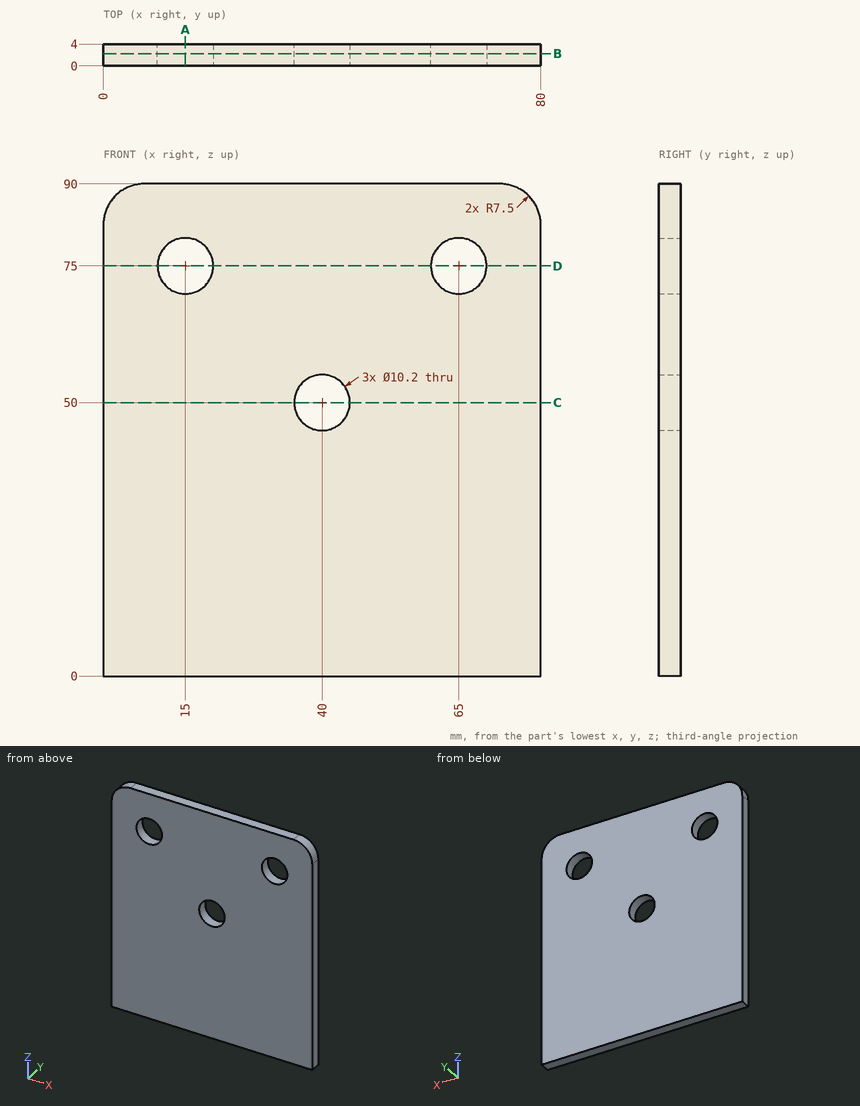
Job drawing, mm, ordinate dimensions from the low corner. One solid piece. Give positions to 0.01 mm unless a question says otherwise; leave off trailing zeros. Order: outer loops, then holes, each group sorted by start corner. A loop starts at its lowest first (then second) coordinate and runs counter-clockwise, first axis right, second up. Notation, with made-up numbers: (80, 69) - (135, 69) arc R23 cw to (135, 85) - close; hole circle Ø5 at (57, 34). An arc over 180 degrees is marked (long way). Return JSON: item names as keys, results as strings.
1) Probe line 1 (Z direction, x = 40, y = 2.1); line 2 (Z direction, x = 65, y = 0.95); line 3 (Z direction, x = 73, y = 0.75). List the from-to ranges inside material, lowest first. Write a range as from..to.
Geometry says:
{"line 1": "0..44.9, 55.1..90", "line 2": "0..69.9, 80.1..90", "line 3": "0..89.98"}
2) Cut at C-C, the plane z = 50. Give the cut face in (x, y).
Geometry says:
{"outline": "(0, 0) - (34.9, 0) - (34.9, 4) - (0, 4) - close; (45.1, 0) - (80, 0) - (80, 4) - (45.1, 4) - close"}
3) Cut at A-A, the plane x = 15. Give the cut face in (y, z), plus the area to 3 significant figures.
Geometry says:
{"outline": "(0, 0) - (4, 0) - (4, 69.9) - (0, 69.9) - close; (0, 80.1) - (4, 80.1) - (4, 90) - (0, 90) - close", "area": "319 mm²"}
4) Flat gauge pin, fed straight in: P1, Ø9, axis at x = 65, z = 75, coming from the -Y side. Where does the tip first touch, or does it go through?
Geometry says:
{"P1": "through"}
5) Cut at D-D, the plane z = 75. Give the cut face in (x, y), plus the area to 3 significant figures.
Geometry says:
{"outline": "(0, 0) - (9.9, 0) - (9.9, 4) - (0, 4) - close; (20.1, 0) - (59.9, 0) - (59.9, 4) - (20.1, 4) - close; (70.1, 0) - (80, 0) - (80, 4) - (70.1, 4) - close", "area": "238 mm²"}
6) Cut at B-B, the plane y = 2.25. Give the cut face in (x, z), plus the area to 3 significant figures.
Geometry says:
{"outline": "(0, 0) - (80, 0) - (80, 82.5) arc R7.5 ccw to (72.5, 90) - (7.5, 90) arc R7.5 ccw to (0, 82.5) - close; hole circle Ø10.2 at (15, 75); hole circle Ø10.2 at (40, 50); hole circle Ø10.2 at (65, 75)", "area": "6,930 mm²"}
